from build123d import *

# Parameters (mm, degrees)
F1_DEPTH = 990.6
F2_R     = 2.75
F3_DEPTH = 25.4


with BuildPart() as f1:
    # F0 (on Front) → F1 (new body)
    with BuildSketch(Plane.XZ):
        with BuildLine():
            ThreePointArc((2.4026723012, -9.7070678278), (7.8748562848, -6.1633301464), (10, 0))
            ThreePointArc((10, 0), (-6.1633301464, 7.8748562848), (-2.4026723012, -9.7070678278))
            Line((-2.4026723012, -9.7070678278), (-2.0930662503, -9.1708144173))
            Line((-2.0930662503, -9.1708144173), (2.0930662503, -9.1708144173))
            Line((2.0930662503, -9.1708144173), (2.4026723012, -9.7070678278))
        make_face()
        with BuildLine():
            Line((-2.0930662503, -9.1708144173), (-2.4026723012, -9.7070678278))
            ThreePointArc((-2.4026723012, -9.7070678278), (0, -10), (2.4026723012, -9.7070678278))
            Line((2.4026723012, -9.7070678278), (2.0930662503, -9.1708144173))
            Line((2.0930662503, -9.1708144173), (-2.0930662503, -9.1708144173))
        make_face()
        with BuildLine():
            ThreePointArc((2.4026723012, -9.7070678278), (0, -10), (-2.4026723012, -9.7070678278))
            Line((-2.4026723012, -9.7070678278), (-9.5, -22))
            Line((-9.5, -22), (-22.5, -22))
            Line((-22.5, -22), (-22.5, -27))
            Line((-22.5, -27), (22.5, -27))
            Line((22.5, -27), (22.5, -22))
            Line((22.5, -22), (9.5, -22))
            Line((9.5, -22), (2.4026723012, -9.7070678278))
        make_face()
    extrude(amount=-F1_DEPTH)

    # F2 (on face) → F3 (cut)
    with BuildSketch(Plane.XY.offset(-22)):
        with Locations((15, 50)):
            Circle(F2_R)
        with Locations((-15, 50)):
            Circle(F2_R)
        with Locations((15, 200)):
            Circle(F2_R)
        with Locations((-15, 200)):
            Circle(F2_R)
        with Locations((15, 350)):
            Circle(F2_R)
        with Locations((-15, 350)):
            Circle(F2_R)
        with Locations((15, 500)):
            Circle(F2_R)
        with Locations((-15, 500)):
            Circle(F2_R)
        with Locations((15, 650)):
            Circle(F2_R)
        with Locations((-15, 650)):
            Circle(F2_R)
        with Locations((15, 800)):
            Circle(F2_R)
        with Locations((-15, 800)):
            Circle(F2_R)
        with Locations((15, 950)):
            Circle(F2_R)
        with Locations((-15, 950)):
            Circle(F2_R)
        with Locations((88.152, 50)):
            Circle(F2_R)
        with Locations((58.152, 50)):
            Circle(F2_R)
        with Locations((88.152, 200)):
            Circle(F2_R)
        with Locations((58.152, 200)):
            Circle(F2_R)
        with Locations((88.152, 350)):
            Circle(F2_R)
        with Locations((58.152, 350)):
            Circle(F2_R)
        with Locations((88.152, 500)):
            Circle(F2_R)
        with Locations((58.152, 500)):
            Circle(F2_R)
        with Locations((88.152, 650)):
            Circle(F2_R)
        with Locations((58.152, 650)):
            Circle(F2_R)
        with Locations((88.152, 800)):
            Circle(F2_R)
        with Locations((58.152, 800)):
            Circle(F2_R)
        with Locations((88.152, 950)):
            Circle(F2_R)
        with Locations((58.152, 950)):
            Circle(F2_R)
        with Locations((161.304, 50)):
            Circle(F2_R)
        with Locations((131.304, 50)):
            Circle(F2_R)
        with Locations((161.304, 200)):
            Circle(F2_R)
        with Locations((131.304, 200)):
            Circle(F2_R)
        with Locations((161.304, 350)):
            Circle(F2_R)
        with Locations((131.304, 350)):
            Circle(F2_R)
        with Locations((161.304, 500)):
            Circle(F2_R)
        with Locations((131.304, 500)):
            Circle(F2_R)
        with Locations((161.304, 650)):
            Circle(F2_R)
        with Locations((131.304, 650)):
            Circle(F2_R)
        with Locations((161.304, 800)):
            Circle(F2_R)
        with Locations((131.304, 800)):
            Circle(F2_R)
        with Locations((161.304, 950)):
            Circle(F2_R)
        with Locations((131.304, 950)):
            Circle(F2_R)
    extrude(amount=-F3_DEPTH, mode=Mode.SUBTRACT)


solid = f1.part
Part model, mm, in its own coordinate system. Coordinates: 2 decimals unless noted, no trailing zeros. Write each loop counter-clockwise with the first axis right and the second up, starting at its lowest first coordinate (ties: lowest second). Pieces come first, ordered by that corner, then holes. Notation, with made-up numbers: M 64.25,-18.75 L 78.25,-18.75 A13 ccw 78.25,-11.75 Z; hole C -38.75,-13 d2. An arc over 180 degrees is marked long. Return JSON: item names as keys, results as strings.
1. Flat gauge pins, fed straight in: pin 1 Ø9 at (x, y) = (-15, 50) entering from +Z; pin 2 Ø3 at (y, z) = (725.5, -8) entering from -X; pin 3 Ø3 at (y, z) = (224.5, -19) entering from +X. Where does each tip first touch, or does it go through?
Determined:
{"pin 1": "z = -22", "pin 2": "x = -7.6", "pin 3": "x = 8.63"}
2. Probe L1, parallel to X at y = 350, z = -24.5; L2, parallel to Z at x = 14, y = 543.5; L3, parallel to Z at x = 0, y = 563. List the from-to ranges inside material, lowest first.
Determined:
{"L1": "-22.5 to -17.75, -12.25 to 12.25, 17.75 to 22.5", "L2": "-27 to -22", "L3": "-27 to 10"}
3. Saw through at A-A, the plane y = 85. Write the cut outline in (x, z), then the cut area to 3 significant figures.
Determined:
{"outline": "M -22.5,-27 L 22.5,-27 L 22.5,-22 L 9.5,-22 L 2.4,-9.71 A10 ccw long -2.4,-9.71 L -9.5,-22 L -22.5,-22 Z", "area": "685 mm²"}
